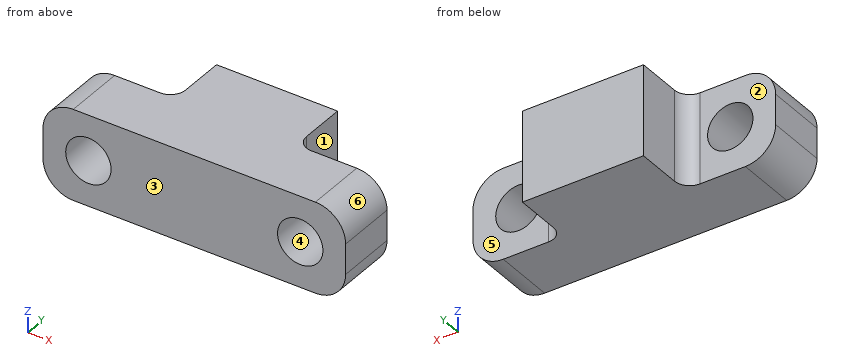
Autodesk Inventor part; units mm, degrees
ref_plane "YZ Plane" through (0, 0, 0) normal (1, 0, 0) x (0, 1, 0)
ref_plane "XZ Plane" through (0, 0, 0) normal (0, 1, 0) x (-1, 0, 0)
ref_plane "XY Plane" through (0, 0, 0) normal (0, 0, 1) x (1, 0, 0)
sketch "Sketch1" plane through (0, 0, 0) normal (0, 0, 1) x (1, 0, 0)
  line L0 (0, 0) -> (0, 12.7)
  line L1 (0, 12.7) -> (19.05, 12.7)
  line L2 (19.05, 12.7) -> (19.05, 25.4)
  line L3 (19.05, 25.4) -> (31.75, 25.4)
  line L4 (31.75, 25.4) -> (31.75, 0)
  line L5 (31.75, 0) -> (0, 0)
  dimension "d0" = 12.7
  dimension "d1" = 31.75
  dimension "d2" = 19.05
  dimension "d3" = 12.7
extrude "Extrusion1" add sketch "Sketch1" along normal blind 19.05
sketch "Sketch2" plane through (0, 12.7, 0) normal (0, 1, 0) x (1, 0, 0)
  line L0 (0, 0) -> (0, -19.05)
  line L1 (0, 0) -> (19.05, 0)
  point P0 (9.525, -9.525)
  dimension "d6" = 9.525
  dimension "d7" = 9.525
hole "Hole1" at (9.525, 12.7, 9.525) direction (0, -1, 0) diameter 9.525 end through all
fillet "Fillet1" radius 6.35 1 edges at (0, 6.35, 19.05)
fillet "Fillet2" radius 6.35 1 edges at (0, 6.35, 0)
mirror "Mirror1" about plane through (31.75, 0, 0) normal (1, 0, 0) of "Extrusion1", "Hole1", "Fillet1", "Fillet2"
fillet "Fillet3" radius 3.175 1 edges at (44.45, 12.7, 9.525)
fillet "Fillet4" radius 3.175 1 edges at (19.05, 12.7, 9.525)
properties part number "Mirror"
Verification items for the finished model (mm, model axes). Face numbers are marked on the shaded views. A direction names the side the tool comes from. Coordinates: 2 decimals unless noted, no trailing zeros. Write each loop counter-clockwise with the first axis right and the second up, starting at its lowest first coordinate (ties: lowest second). Pieces come first, ordered by that corner, then holes. Notation, with made-up numbers: (88.5, 40) - (124.5, 40) arc R31 ccw to (124.5, 72) - close; hole circle Ø3 at (82.25, -22.75). An arc over 180 degrees is marked (long way). One line per question, with ' | ' between items. Start each with the question number.
1. Section check C-C (y = 10.5). Count the separate pieces of the cut face and the enclosed holes in it, plus the area to 3 significant figures.
2. Section check A-A (z = 9.5). Enter the section's corners in (x, y) (3 decimals).
3. Draft check along X on the marked faces 4, 5 and 6. Enter one of: released by +X, released by -X, zero draft, split by the parting line, or undercut.
4. Section check D-D (y = 17.25). Enter the section's corners in (x, z).
5. Material ranges on line 1 along X through (y, z) = (6.25, 5.75); line 2 along X through (y, z) = (9, 6.25); line 3 along Y through (x, z) = (14, 6.5), recorded low to high.
6. Gauge pin test, flat ends, axial feed: P1, Ø10.5, axis at y = 19, z = 12.5, coming from the +X side; P2, Ø1, axis at y = 9.5, z = 14, coming from the -X side; P3, Ø10, axis at x = 11.5, y = 18.5, coming from the +Z side; P4, Ø4, axis at x = 56, z = 14.5, coming from the +Y side. Record the tip position at first contact, or that the pin passes through.
7. Access from +Z, -Z, +X, -X, +Y, -Y to the whole of each face (thin tool, end or side, straight path). Record for the marked faces 1, 2 and 3.
8. Section check B-B (x = 52). Enter the section's corners in (y, z), plus the area to 3 significant figures.
Computed values:
1) separate pieces: 1 | enclosed holes: 2 | area: 1,030 mm²
2) outline: (0, 0) - (4.763, 0) - (4.763, 12.7) - (0, 12.7) - close; (14.287, 0) - (49.213, 0) - (49.213, 12.7) - (47.625, 12.7) arc R3.175 cw to (44.45, 15.875) - (44.45, 25.4) - (19.05, 25.4) - (19.05, 15.875) arc R3.175 cw to (15.875, 12.7) - (14.287, 12.7) - close; (58.737, 0) - (63.5, 0) - (63.5, 12.7) - (58.737, 12.7) - close
3) face 4: undercut | face 5: zero draft | face 6: released by +X
4) outline: (19.05, 0) - (44.45, 0) - (44.45, 19.05) - (19.05, 19.05) - close
5) line 1: 0.03 to 6.62, 12.43 to 51.07, 56.88 to 63.47 | line 2: 0 to 6.07, 12.98 to 50.52, 57.43 to 63.5 | line 3: 0 to 12.7
6) P1: x = 45.27 | P2: x = 0.05 | P3: through | P4: y = 12.7
7) face 1: +Z, -Z, +X, +Y | face 2: +Z, -Z, -X, +Y | face 3: +Z, -Z, +X, -X, -Y
8) outline: (0, 0) - (12.7, 0) - (12.7, 5.19) - (0, 5.19) - close; (0, 13.86) - (12.7, 13.86) - (12.7, 19.05) - (0, 19.05) - close | area: 132 mm²
